from build123d import *

# Parameters (mm, degrees)
SKETCH_W        = 10
SKETCH_H        = 20
PAD_DEPTH       = 16
SKETCH001_W     = 10
SKETCH001_H     = 17
POCKET_DEPTH    = 4.5
SKETCH002_W     = 10
SKETCH002_H     = 9.4
POCKET001_DEPTH = 6.5
SKETCH003_R     = 1.7
POCKET002_DEPTH = 5
SKETCH004_R     = 2.8
POCKET003_DEPTH = 3
FILLET_R        = 1
FILLET001_R     = 1


with BuildPart() as part:
    # Sketch → Pad (new body)
    with BuildSketch(Plane.XY):
        Rectangle(SKETCH_W, SKETCH_H)
    extrude(amount=PAD_DEPTH)

    # Sketch001 (on Face6 of Pad) → Pocket (cut)
    with BuildSketch(Plane.XY.offset(16)):
        with Locations((0, -1.5)):
            Rectangle(SKETCH001_W, SKETCH001_H)
    extrude(amount=-POCKET_DEPTH, mode=Mode.SUBTRACT)

    # Sketch002 (on Face4 of Pocket) → Pocket001 (cut)
    with BuildSketch(Plane(origin=(0, 0, 0), x_dir=(1, 0, 0), z_dir=(0, 0, -1))):
        Rectangle(SKETCH002_W, SKETCH002_H)
    extrude(amount=-POCKET001_DEPTH, mode=Mode.SUBTRACT)

    # Sketch003 (on Face8 of Pocket001) → Pocket002 (cut)
    with BuildSketch(Plane(origin=(0, 0, 6.5), x_dir=(1, 0, 0), z_dir=(0, 0, -1))):
        with Locations((-0.5, 0)):
            Circle(SKETCH003_R)
    extrude(amount=-POCKET002_DEPTH, mode=Mode.SUBTRACT)

    # Sketch004 (on Face11 of Pocket002) → Pocket003 (cut)
    with BuildSketch(Plane.XY.offset(11.5)):
        with Locations((-0.5, 0)):
            Circle(SKETCH004_R)
    extrude(amount=-POCKET003_DEPTH, mode=Mode.SUBTRACT)

    # Fillet
    fillet_edges = [part.edges().sort_by_distance(p)[0] for p in [
        (0, -4.7, 0),
    ]]
    fillet(fillet_edges, radius=FILLET_R)

    # Fillet001
    fillet001_edges = [part.edges().sort_by_distance(p)[0] for p in [
        (0, 4.7, 0),
    ]]
    fillet(fillet001_edges, radius=FILLET001_R)


solid = part.part
Check sheet for the modelled part. Datum: model origin and axes. Units: mm. A direction names the side the tool comes from. Give positions to 0.01 mm unless a question says otherwise; leave off trailing zeros. Order: outer loops, then holes, each group sorted by start corner. A loop starts at its lowest first (then second) coordinate and runs counter-clockwise, first axis right, second up. Notation, with made-up numbers: (15.25, 0) - (31.25, 0) arc R15 cw to (31.25, 17) - close; hole circle Ø3 at (29.5, 51.5). An arc over 180 degrees is marked (long way). Answer as CSV lines item,"result".
1. Section check A-A (y = 0). Record the boundary of the cut face in (x, z).
Result sheet:
outline,"(-5, 6.5) - (-2.2, 6.5) - (-2.2, 8.5) - (-3.3, 8.5) - (-3.3, 11.5) - (-5, 11.5) - close; (1.2, 6.5) - (5, 6.5) - (5, 11.5) - (2.3, 11.5) - (2.3, 8.5) - (1.2, 8.5) - close"
2. Scan lines: probe 1 along Y at (x, z) = (-0.5, 10.3); probe 2 along X at (y, z) = (0, 7.8); probe 3 along Z at (x, y) = (-0.25, -3.5). Record each from-to range of solid material in increasing order. Write a range as from..to.
Result sheet:
probe 1,"-10..-2.8, 2.8..10"
probe 2,"-5..-2.2, 1.2..5"
probe 3,"6.5..11.5"
3. Go/stop test with flat-tipped pins: P1, Ø4, axis at x = 3.5, y = -0.5, coming from the +Z side; P2, Ø1.3, axis at x = 1, z = 13, coming from the -Y side; P3, Ø4.5, axis at x = 1.5, y = 0, coming from the -Z side. Record where each tip stops, or that it passes through.
Result sheet:
P1,"z = 11.5"
P2,"y = 7"
P3,"z = 6.5"
4. Section check C-C (x = -0.5). Record the boundary of the cut face in (y, z), then the cut area to 3 significant figures.
Result sheet:
outline,"(-10, 0) - (-5.7, 0) arc R1 ccw to (-4.7, 1) - (-4.7, 6.5) - (-1.7, 6.5) - (-1.7, 8.5) - (-2.8, 8.5) - (-2.8, 11.5) - (-10, 11.5) - close; (1.7, 6.5) - (4.7, 6.5) - (4.7, 1) arc R1 ccw to (5.7, 0) - (10, 0) - (10, 16) - (7, 16) - (7, 11.5) - (2.8, 11.5) - (2.8, 8.5) - (1.7, 8.5) - close"
area,"158 mm²"
5. Mould release check, pull along X, two halves, no side actions. Record for faces 5 (the face through (-5, 0, 8)), 6 (the face through (0, -3, 11.5)), 7 (the face through (-1, -2, 8.5)): released by +X, released by -X, zero draft, split by the parting line, or undercut.
Result sheet:
face 5,"released by -X"
face 6,"zero draft"
face 7,"undercut"
6. Section check D-D (x = 3.5). Record the boundary of the cut face in (y, z).
Result sheet:
outline,"(-10, 0) - (-5.7, 0) arc R1 ccw to (-4.7, 1) - (-4.7, 6.5) - (4.7, 6.5) - (4.7, 1) arc R1 ccw to (5.7, 0) - (10, 0) - (10, 16) - (7, 16) - (7, 11.5) - (-10, 11.5) - close"
7. Section check B-B (z = 4.25). Record the boundary of the cut face in (x, y).
Result sheet:
outline,"(-5, -10) - (5, -10) - (5, -4.7) - (-5, -4.7) - close; (-5, 4.7) - (5, 4.7) - (5, 10) - (-5, 10) - close"
8. Tool access check on faces 1 (the face through (0, 7, 14)), 2 (the face through (0, 10, 8)), 3 (the face through (-3.3, 0.1, 10)), 4 (the face through (0.07, -5.001, 0.285)). Record the directions out of +Z, -Z, +X, -X, +Y, -Y that give a thin tool (end or side, any length) a straight path to the whole face; none if there is none.
Result sheet:
face 1,"+Z, +X, -X, -Y"
face 2,"+Z, -Z, +X, -X, +Y"
face 3,"+Z"
face 4,"-Z, +X, -X"
